Check sheet for the drawn part. Datum: minimum x, y, z corner. Units: mm. Give positions to 0.01 mm unless a question says otherwise; leave off trailing zeros. Order: outer loops, then holes, each group sorted by start corner. A loop starts at its lowest first (then second) coordinate and runs counter-clockwise, first axis right, second up. Notation, with made-up numbers: (-20.5, 75.25) -> (16.5, 75.25) arc R20 ccw to (16.5, 91.25) -> close; hole circle Ø2 at (-5, -21). An arc over 180 degrees is marked (long way). Answer in a Markdown table with one row per item. Add a question column.
(1) Go/stop test with a flat-tipped pin: pin 1 (3 mm diameter, centred on x = 148.5, z = 81.5, fed in from -Y). Record where the tip stops, or that it passes through.
(2) Cross-section at B-B (z = 80). Record the cut outline in (x, y).
(3) Cross-section at A-A (y = 150). Record the cut outline in (x, z), then the cut area to 3 significant figures.
(4) Thickness scan on L1, parallel to X at y = 5, z = 80; L2, parallel to Y at x = 319, z = 80. Record the ranges inside material, lowest first. Write a range as [from, to].
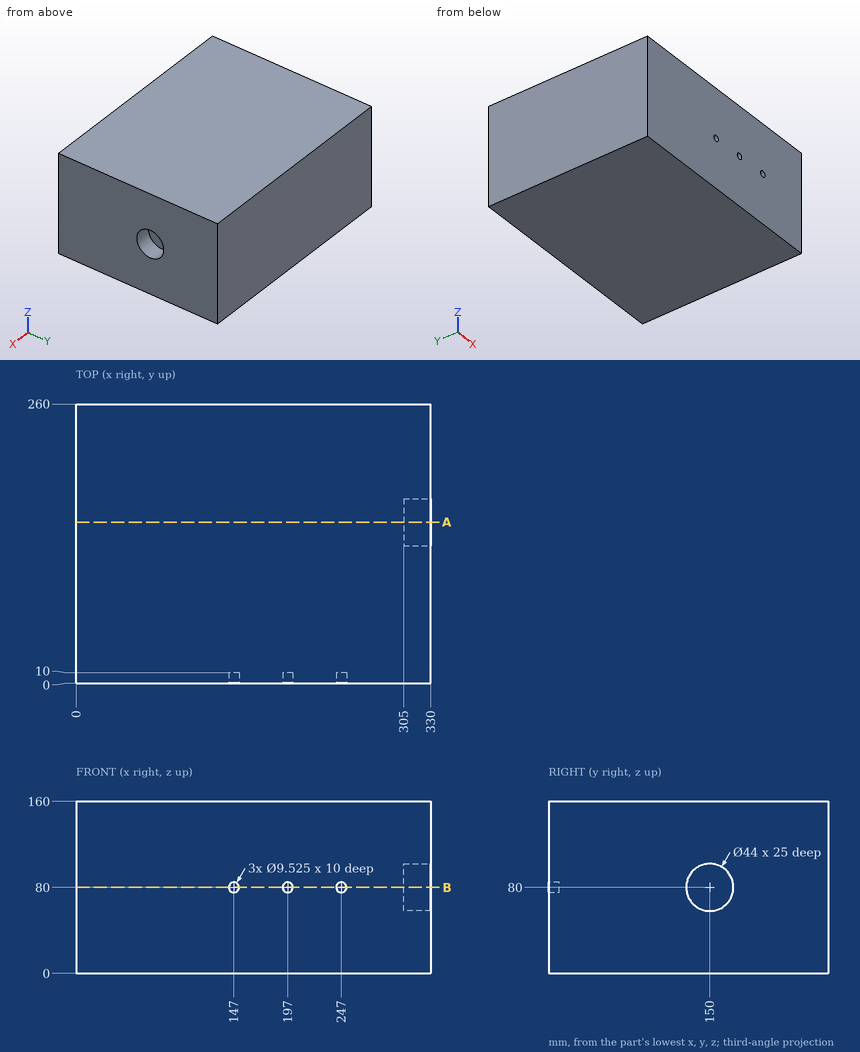
Answer below:
| question | item | result |
|---|---|---|
| 1 | pin 1 | stops at y = 10 |
| 2 | outline | (0, 0) -> (142.24, 0) -> (142.24, 10) -> (151.76, 10) -> (151.76, 0) -> (192.24, 0) -> (192.24, 10) -> (201.76, 10) -> (201.76, 0) -> (242.24, 0) -> (242.24, 10) -> (251.76, 10) -> (251.76, 0) -> (330, 0) -> (330, 128) -> (305, 128) -> (305, 172) -> (330, 172) -> (330, 260) -> (0, 260) -> close |
| 3 | outline | (0, 0) -> (330, 0) -> (330, 58) -> (305, 58) -> (305, 102) -> (330, 102) -> (330, 160) -> (0, 160) -> close |
| 3 | area | 51,700 mm² |
| 4 | L1 | x = [0, 142.24], [151.76, 192.24], [201.76, 242.24], [251.76, 330] |
| 4 | L2 | y = [0, 128], [172, 260] |
